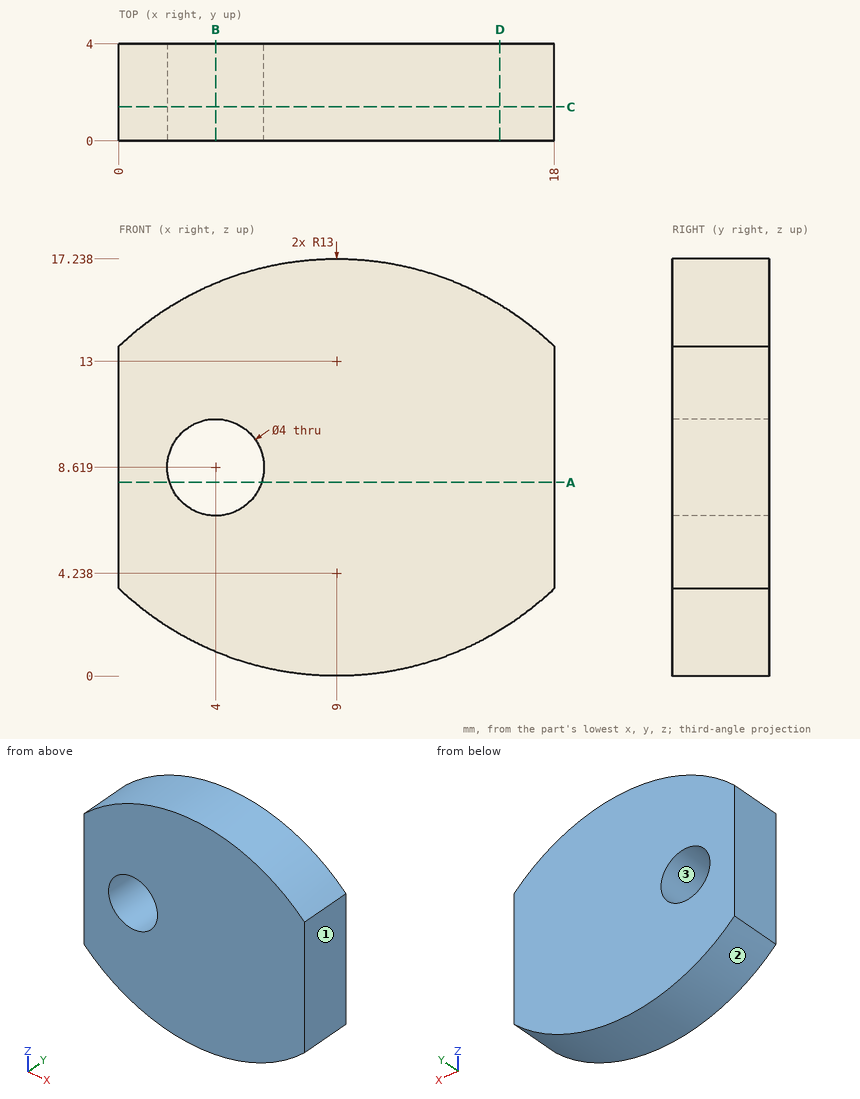
Geometry: see drawing. Coordinates: mm, zero at the bounding-box minimum. Coordinates: 2 decimals unless noted, no trailing zeros. Order: outer loops, then holes, each group sorted by start corner. A loop starts at its lowest first (then second) coordinate and runs counter-clockwise, first axis right, second up. Notation, with made-up numbers: M 28.25,47 L 43.25,47 A26 cw 43.25,84 Z; hole C -33,-25.5 d4. An arc over 180 degrees is marked long. Answer in a Markdown table with one row per item. Add a question column.
Q1. Section query D-D on x = 15.75. Return the cut outline in (y, z).
Q2. Line query: L1, parallel to Z at x = 8.75, y = 0.6; L2, parallel to Z at x = 2.75, y = 3.1; L3, parallel to Z at x = 4.25, y = 2.15 (1 decimal). Output: solid intervals per line, ascending.
Q3. Section query A-A on z = 8. Return the cut outline in (x, y).
Q4. Section query B-B on x = 4. Return the cut outline in (y, z).
Q5. Contact query for a flat-ended pin moving along its axis: P1, Ø1.5, axis at x = 7.5, z = 14.5, coming from the -Y side. Output: stop coordinate, or through.
Q6. Mould query, pull axis Z, two halves, no side actions, for the marked faces 1, 2 and 3. Classes: released by +Z, released by -Z, zero draft, split by the parting line, or undercut.
Q7. Section query C-C on y = 1.4. Return the cut outline in (x, z), and give its area (3 significant figures).
Completed:
| question | item | result |
|---|---|---|
| 1 | outline | M 0,1.89 L 4,1.89 L 4,15.35 L 0,15.35 Z |
| 2 | L1 | z = 0 to 17.24 |
| 2 | L2 | z = 1.6 to 7.06, 10.18 to 15.64 |
| 2 | L3 | z = 0.9 to 6.6, 10.6 to 16.3 |
| 3 | outline | M 0,0 L 2.1,0 L 2.1,4 L 0,4 Z; M 5.9,0 L 18,0 L 18,4 L 5.9,4 Z |
| 4 | outline | M 0,1 L 4,1 L 4,6.62 L 0,6.62 Z; M 0,10.62 L 4,10.62 L 4,16.24 L 0,16.24 Z |
| 5 | P1 | stops at y = 0 |
| 6 | face 1 | zero draft |
| 6 | face 2 | released by -Z |
| 6 | face 3 | undercut |
| 7 | outline | M 0,3.62 A13 ccw 18,3.62 L 18,13.62 A13 ccw 0,13.62 Z; hole C 4,8.62 d4 |
| 7 | area | 257 mm2 |
